Here's how the part is built. I have some questions about the finished solid (model axes, mm). A direction names the side the tool comes from. Round coordinates to 2 decimals unless told otherwise and drop trailing zeros. Loops run counter-clockwise (first coordinate to the right, second up) from the corner with the lowest first, then second, coordinate; pieces in that order, holes last. Notation, with made-up numbers: (41.5, 7) - (97.5, 7) arc R5 cw to (97.5, 11) - close; hole circle Ø8 at (3, 69). An arc over 180 degrees is marked (long way). Answer as a JSON object with one key per item and string values. Group by question number.
1) If we mould it in two halves opening along X, with no side actions, what happens to faces 1 (the face through (0.945, -21, 5)), 2 (the face through (-15.25, 1, 0)), 3 (the face through (0, -8, 10.75))? For each: pulls with the +X half, pulls with the -X half, needs draft (parallel to the pull), parting line crosses it, or undercut.
2) Will these pins go through, and if not, where does the flat tip stop? P1, Ø1.5, axis at x = -1.5, y = -16, coming from the -Z side; P2, Ø0.8, axis at x = 9, y = -21, coming from the -Z side; P3, Ø1.5, axis at x = -6, z = -9.5, coming from the -Y side; P4, Ø12, axis at x = 10, z = -5, coming from the +Y side.
3) I want a section at B-B, the plane x = 3.5. Please give me the cut outline in (y, z), then the cut area to 3 significant figures.
4) If I drill on line 1 along X through (y, z) = (-20.5, -4.25); line 2 along Z through (x, y) = (0, -23); line 3 along Z through (x, y) = (-2.5, -3.5), over which ranges is the centre line in solid material (lowest first)? Write a range as [from, to].
5) I want a section at C-C, the plane y = -10.5. Please give me the cut outline in (x, z), then the cut area to 4 significant figures.
6) I want a section at D-D, the plane z = -10.25. Please give me the cut outline in (x, y).
7) I want a section at A-A, the plane z = 1.75. Please give me the cut outline in (x, y).
8) Which directions (+Z, -Z, +X, -X, +Y, -Y) give clear straight access to the entire face, cutting with the end or side of a thin tool? Please do faces 4 (the face through (9, -21, -7.167)), 5 (the face through (0, -21, 7.674)), 6 (the face through (10.018, -21, -4)).
from build123d import *

# Parameters (mm, degrees)
SKETCH_1_W      = 30.5
SKETCH_1_H      = 25
EXTRUDE_1_DEPTH = 2
SKETCH_2_W      = 29
SKETCH_2_H      = 21.5
EXTRUDE_2_DEPTH = 16
SKETCH_3_W      = 1.802565081
SKETCH_3_H      = 5.167353231
SKETCH_3_H_2    = 6.008550268
SKETCH_3_W_2    = 1.682394075
SKETCH_3_H_3    = 6.008550269
SKETCH_3_W_3    = 1.622308572
EXTRUDE_3_DEPTH = 9.6
EXTRUDE_4_DEPTH = 9.25


with BuildPart() as part:
    # 草图1 → 凸台-拉伸1 (new body)
    with BuildSketch(Plane(origin=(0, 0, 0), x_dir=(1, 0, 0), z_dir=(0, 1, 0))):
        Rectangle(SKETCH_1_W, SKETCH_1_H)
    extrude(amount=EXTRUDE_1_DEPTH)

    # 草图2 → 凸台-拉伸2 (add)
    with BuildSketch(Plane.XZ):
        Rectangle(SKETCH_2_W, SKETCH_2_H)
    extrude(amount=EXTRUDE_2_DEPTH)

    # 草图3 → 凸台-拉伸3 (add)
    with BuildSketch(Plane.XZ.offset(16)):
        with Locations((-9.810401899, 5.210817025)):
            Rectangle(SKETCH_3_W, SKETCH_3_H)
        with Locations((-9.810401899, -4.222606897)):
            Rectangle(SKETCH_3_W, SKETCH_3_H_2)
        with Locations((0.103706044, 5.09064602)):
            Rectangle(SKETCH_3_W_2, SKETCH_3_H)
        with Locations((0.103706044, -4.342777902)):
            Rectangle(SKETCH_3_W_2, SKETCH_3_H_3)
        with Locations((9.206659702, 5.270902528)):
            Rectangle(SKETCH_3_W_3, SKETCH_3_H)
        with Locations((9.206659702, -4.162521395)):
            Rectangle(SKETCH_3_W_3, SKETCH_3_H_3)
    extrude(amount=EXTRUDE_3_DEPTH)

    # 草图4 → 凸台-拉伸4 (add, symmetric)
    with BuildSketch(Plane.XY):
        with BuildLine():
            Line((10.382594104, 2), (-10.382594104, 2))
            Line((-10.382594104, 2), (-9.22822883, 6.460566864))
            ThreePointArc((-9.22822883, 6.460566864), (-4.784721142, 4.572616283), (0, 3.927975641))
            ThreePointArc((0, 3.927975641), (4.784721142, 4.572616283), (9.22822883, 6.460566864))
            Line((9.22822883, 6.460566864), (10.382594104, 2))
        make_face()
    extrude(amount=EXTRUDE_4_DEPTH, both=True)


solid = part.part
Outcome:
{
 "1": {"face 1": "undercut", "face 2": "pulls with the -X half", "face 3": "needs draft"},
 "2": {"P1": "z = -10.75", "P2": "z = -7.17", "P3": "y = -16", "P4": "y = 6.46"},
 "3": {"outline": "(-16, -10.75) - (0, -10.75) - (0, -12.5) - (2, -12.5) - (2, -9.25) - (4.27, -9.25) - (4.27, 9.25) - (2, 9.25) - (2, 12.5) - (0, 12.5) - (0, 10.75) - (-16, 10.75) - close", "area": "436 mm^2"},
 "4": {"line 1": "[-10.71, -8.91], [-0.74, 0.94], [8.4, 10.02]", "line 2": "[-7.35, -1.34], [2.51, 7.67]", "line 3": "[-10.75, 10.75]"},
 "5": {"outline": "(-14.5, -10.75) - (14.5, -10.75) - (14.5, 10.75) - (-14.5, 10.75) - close", "area": "623.5 mm^2"},
 "6": {"outline": "(-15.25, 0) - (-14.5, 0) - (-14.5, -16) - (14.5, -16) - (14.5, 0) - (15.25, 0) - (15.25, 2) - (-15.25, 2) - close"},
 "7": {"outline": "(-15.25, 0) - (-14.5, 0) - (-14.5, -16) - (14.5, -16) - (14.5, 0) - (15.25, 0) - (15.25, 2) - (10.38, 2) - (9.23, 6.46) arc R18.08 cw to (-9.23, 6.46) - (-10.38, 2) - (-15.25, 2) - close"},
 "8": {"face 4": "-Z, +X, -Y", "face 5": "+Z, -Y", "face 6": "+Z, -Z, +X, -Y"}
}
